from build123d import *

# Parameters (mm, degrees)
BOSS_EXTRUDE1_START = 9.9
BOSS_EXTRUDE1_DEPTH = 56.9
SKETCH3_W           = 15
SKETCH3_H           = 3
SKETCH3_W_2         = 4.7
SKETCH3_H_2         = 2
BOSS_EXTRUDE2_DEPTH = 3.5
FILLET1_R           = 0.5


with BuildPart() as part:
    # Sketch1 → Boss-Extrude1 (new body)
    with BuildSketch(Plane(origin=(0, 0, 0), x_dir=(0, 0, -1), z_dir=(1, 0, 0)).offset(BOSS_EXTRUDE1_START)):
        Polygon((3.6, -4.5), (3.6, 4.9), (1.6, 4.9), (1.6, -2.5), (-1.4, -2.5), (-1.4, -4.5), align=None)
    extrude(amount=BOSS_EXTRUDE1_DEPTH)

    # Sketch3 → Boss-Extrude2 (add)
    with BuildSketch(Plane(origin=(0, -2.5, 0), x_dir=(1, 0, 0), z_dir=(0, 1, 0))):
        Polygon((32.9, -1.4), (17.9, -1.4), (17.9, -9.4), (9.9, -9.4), (9.9, -15.1), (32.9, -15.1), align=None)
        Polygon((58.8, -1.4), (54.1, -1.4), (54.1, -15.1), (66.8, -15.1), (66.8, -7.4), (58.8, -7.4), align=None)
        with Locations((25.4, 0.1)):
            Rectangle(SKETCH3_W, SKETCH3_H)
        with Locations((56.45, 0.1)):
            Rectangle(SKETCH3_W_2, SKETCH3_H)
        with Locations((25.4, 2.6)):
            Rectangle(SKETCH3_W, SKETCH3_H_2)
        with Locations((56.45, 2.6)):
            Rectangle(SKETCH3_W_2, SKETCH3_H_2)
    extrude(amount=-BOSS_EXTRUDE2_DEPTH)

    # Fillet1
    fillet1_edges = [part.edges().sort_by_distance(p)[0] for p in [
        (9.9, -4.5, -1.1),
        (9.9, -3.5, 1.4),
        (13.9, -4.5, -3.6),
        (13.9, -4.5, 1.4),
        (9.9, 4.9, -2.6),
        (66.8, -4.5, -1.1),
        (9.9, -6, 12.25),
        (62.8, -4.5, 1.4),
        (9.9, -4.25, 15.1),
        (21.4, -6, 15.1),
        (32.9, -4.25, 15.1),
        (32.9, -5.25, -3.6),
        (32.9, -4.5, -1.1),
        (32.9, -3.5, 1.4),
        (32.9, -6, 5.75),
        (17.9, -5.25, -3.6),
        (25.4, -6, -3.6),
        (66.8, -3.5, 1.4),
        (17.9, -3.5, 1.4),
        (17.9, -4.5, -1.1),
        (17.9, -6, 2.9),
        (17.9, -4.25, 9.4),
        (13.9, -6, 9.4),
        (9.9, -4.25, 9.4),
        (38.35, -2.5, -1.6),
        (66.8, 4.9, -2.6),
        (38.35, 4.9, -3.6),
        (66.8, 0.2, -3.6),
        (62.8, -4.5, -3.6),
        (43.5, -4.5, -3.6),
        (43.5, -4.5, 1.4),
        (66.8, -4.25, 7.4),
        (60.45, -6, 15.1),
        (66.8, -4.25, 15.1),
        (54.1, -3.5, 1.4),
        (54.1, -4.5, -1.1),
        (54.1, -6, 5.75),
        (54.1, -4.25, 15.1),
        (54.1, -5.25, -3.6),
        (56.45, -6, -3.6),
        (58.8, -5.25, -3.6),
        (58.8, -4.5, -1.1),
        (58.8, -3.5, 1.4),
        (58.8, -6, 1.9),
        (58.8, -4.25, 7.4),
        (62.8, -6, 7.4),
        (66.8, -6, 11.25),
        (9.9, 0.2, -3.6),
    ]]
    fillet(fillet1_edges, radius=FILLET1_R)


solid = part.part
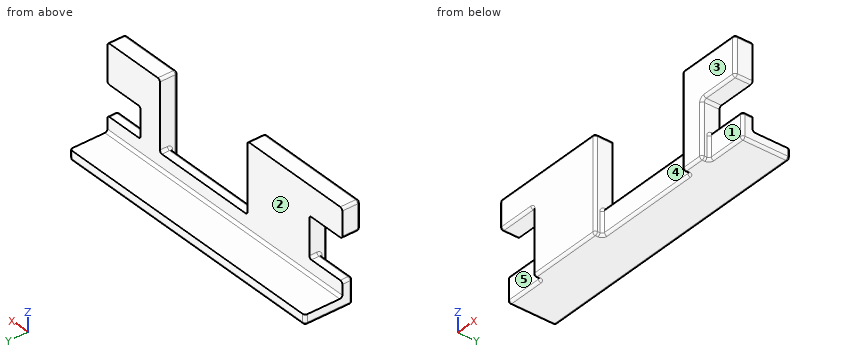
Can you work these out from the model? Positions are in its coordinate system, mm. Face numbers are marked on the shaded views. A direction names the side the tool comes from. Coordinates: 2 decimals unless noted, no trailing zeros. Loops run counter-clockwise (first coordinate to the right, second up) from the corner with the lowest first, then second, coordinate; pieces in that order, holes last. Notation, with made-up numbers: (53.5, -33.75) - (89.5, -33.75) arc R21 ccw to (89.5, -27.75) - close; hole circle Ø4 at (32.5, -9). An arc over 180 degrees is marked (long way). Put each result on its own line as item: value. Start each with the question number.
Item 1: Which directions (+Z, -Z, +X, -X, +Y, -Y) give clear straight access to the entire face, cutting with the end or side of a thin tool? Please do the marked faces 1, 2 and 3.
Item 2: Suppose I cut it at A-A (x = 61.5). Please give me the cut outline in (y, z).
Item 3: Suppose I cut it at B-B (z = 6). Please give me the cut outline in (x, y).
Item 4: For pin 1 (3 mm diameter, centred on y = 2, z = 0, fed in from +X); pin 2 (5.5 mm diameter, centred on x = 37, y = 0.5, fed in from +Z); pin 3 (4.5 mm diameter, centred on x = 42.5, z = -1, fed in from -Y); pin 4 (1.5 mm diameter, centred on y = -4, z = 2, fed in from -X), each with a flat end and sliding along its axis, tell me the tip position at first contact or that it passes through.
Item 5: If we mould it in two halves opening along X, with no side actions, what happens to the marked faces 4 and 5? For each: +X half, -X half, draft (parallel to the pull), parting line (faces both ways), or undercut.
Item 6: If I drill on line 1 along X through (y, z) = (-5.5, 3.25); line 2 along Y through (x, z) = (57, 0.25); line 3 along Z through (x, y) = (58.5, 2), over which ranges is the centre line in solid material (lowest first)?
Item 7: Suppose I cut it at D-D (x = 23.5). Please give me the cut outline in (y, z).
Here are the results:
1. face 1: -Z, +X, -Y
1. face 2: +Z, +X, -X, +Y
1. face 3: +Z, -Z, +X, -X, -Y
2. outline: (-6, 7.9) arc R0.5 ccw to (-5.5, 7.4) - (-2.5, 7.4) - (-2.5, 15.1) - (-5.5, 15.1) arc R0.5 ccw to (-6, 14.6) - close; (-4.5, -3.1) arc R0.5 ccw to (-4, -3.6) - (4.4, -3.6) arc R0.5 ccw to (4.9, -3.1) - (4.9, -1.6) - (-2, -1.6) arc R0.5 cw to (-2.5, -1.1) - (-2.5, 1.4) - (-4, 1.4) arc R0.5 ccw to (-4.5, 0.9) - close
3. outline: (17.9, -5.5) arc R0.5 ccw to (18.4, -6) - (32.4, -6) arc R0.5 ccw to (32.9, -5.5) - (32.9, -2.5) - (17.9, -2.5) - close; (54.1, -5.5) arc R0.5 ccw to (54.6, -6) - (58.3, -6) arc R0.5 ccw to (58.8, -5.5) - (58.8, -2.5) - (54.1, -2.5) - close
4. pin 1: through
4. pin 2: z = -1.53
4. pin 3: y = -4.5
4. pin 4: x = 10.04
5. face 4: undercut
5. face 5: draft
6. line 1: 17.9 to 32.9, 54.1 to 58.8
6. line 2: -6 to -2.5
6. line 3: -3.6 to -1.6
7. outline: (-6, -3.1) arc R0.5 ccw to (-5.5, -3.6) - (4.4, -3.6) arc R0.5 ccw to (4.9, -3.1) - (4.9, -1.6) - (-2, -1.6) arc R0.5 cw to (-2.5, -1.1) - (-2.5, 15.1) - (-5.5, 15.1) arc R0.5 ccw to (-6, 14.6) - close
